Source: CAD feature listing. Evaluate the final solid. Frame: model axes, mm. Face numbers are marked on the shaded views. A direction names the side the tool comes from. Round coordinates to 2 decimals unless told otherwise and drop trailing zeros. Loops run counter-clockwise (first coordinate to the right, second up) from the corner with the lowest first, then second, coordinate; pieces in that order, holes last.
Item 1: Access query for the marked faces 1 and 2. Directions: +Z, -Z, +X, -X, +Y, -Y. A direction counts if a zero-diameter tool reaches every point of the face in a straight line with its end or side. Return the directions, or none.
Item 2: First-contact query: P1, Ø1, axis at x = -1, z = -19.5, coming from the -Y side; P2, Ø0.5, axis at y = 0, z = -0.5, coming from the -X side; P3, Ø4, axis at y = 2, z = -8.5, coming from the +X side. Flat tips, straight axial feed; report the tip coordinate or a pass-through.
Item 3: Ray query, L1, parallel to X at y = 1, z = -7.75; L2, parallel to Z at x = 2.25, y = 1; L3, parallel to Y at x = 1.25, z = -12.75. Return the intervals inside material, ascending.
Item 4: Section query A-A on x = 0. Return loops of the section in (y, z), then the cut area to 3 significant figures.
Item 5: Section query C-C on z = -12.75. Return loops of the section in (x, y), then the cut area to 3 significant figures.
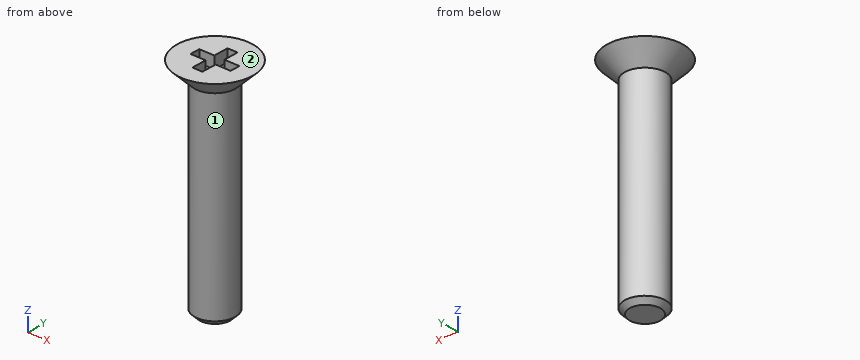
Solid Edge part; units mm, degrees
sketch "Sketch1" plane through (0, 0, 0) normal (0, -1, 0) x (1, 0, 0)
  line L0 (0, 0) -> (3.75, 0)
  line L1 (3.75, 0) -> (2, -1.75)
  line L2 (2, -1.75) -> (2, -21.75)
  line L3 (2, -21.75) -> (0, -21.75)
  dimension "D1" = 2
revolve "RevolvedProtrusion1" add sketch "Sketch1" angle 360 about axis through (0, 0, -21.75) along (0, 0, 1)
chamfer "Chamfer_1" distance 0.5 angle 45 1 edges at (-2, 0, -21.75)
sketch "Sketch2" plane through (0, 0, 0) normal (0, 0, 1) x (0, 1, 0)
  line L0 (0.5, -0.5) -> (2, -0.5)
  line L1 (2, -0.5) -> (2, 0.5)
  line L2 (2, 0.5) -> (0.5, 0.5)
  line L3 (0.5, 2) -> (0.5, 0.5)
  line L4 (-0.5, 2) -> (0.5, 2)
  line L5 (-0.5, 0.5) -> (-0.5, 2)
  line L6 (-0.5, 0.5) -> (-2, 0.5)
  line L7 (-2, 0.5) -> (-2, -0.5)
  line L8 (-2, -0.5) -> (-0.5, -0.5)
  line L9 (-0.5, -2) -> (-0.5, -0.5)
  line L10 (0.5, -2) -> (-0.5, -2)
  line L11 (0.5, -0.5) -> (0.5, -2)
  dimension "D1" = 0.5
extrude "ExtrudedCutout_1" cut sketch "Sketch2" against normal blind 1.2
cosmetic_thread "Thread1"
properties material "Stainless steel"
Data:
1. face 1: -Z
1. face 2: +Z, +X, -X, +Y, -Y
2. P1: stops at y = -1.94
2. P2: stops at x = -3.5
2. P3: stops at x = 2
3. L1: x = -1.73 to 1.73
3. L2: z = -1.29 to 0
3. L3: y = -1.56 to 1.56
4. outline: (-3.75, 0) - (-2, -1.75) - (-2, -21.25) - (-1.5, -21.75) - (1.5, -21.75) - (2, -21.25) - (2, -1.75) - (3.75, 0) - (2, 0) - (2, -1.2) - (-2, -1.2) - (-2, 0) - close
4. area: 85.0 mm2
5. outline: circle Ø4 at (0, 0)
5. area: 12.6 mm2
